```python
from build123d import *

# Parameters (mm, degrees)
BOSS_EXTRUDE1_DEPTH  = 6.604
MOVE_FACE1_DEPTH     = 6.604
MOVE_FACE1_2_DEPTH   = 6.604
BOSS_EXTRUDE2_DEPTH  = 21.59
BOSS_EXTRUDE3_REACH  = 135.651
FILLET1_R            = 12.7
BOSS_EXTRUDE4_DEPTH  = 4.0259
MIRROR3_COPY_1_DEPTH = 4.0259
SKETCH13_R           = 6.35
CUT_EXTRUDE1_DEPTH   = 110.931012164
SKETCH9_R            = 47.625
SKETCH9_R_2          = 43.434
BOSS_EXTRUDE7_DEPTH  = 1.27
CUT_EXTRUDE2_START   = -5.08
SKETCH15_R           = 43.434
CUT_EXTRUDE2_DEPTH   = 5.08
SKETCH16_R           = 15.24
CUT_EXTRUDE3_DEPTH   = 2.54
SKETCH17_R           = 15.24
BOSS_EXTRUDE8_DEPTH  = 11.2395
SKETCH18_R           = 12.7
CUT_EXTRUDE4_DEPTH   = 6.35


# Read off the part's stored shape, not the designer's step: Move Face1
with BuildPart() as part:
    # Sketch1 → Boss-Extrude1 (new body)
    with BuildSketch(Plane(origin=(0, 0, 0), x_dir=(1, 0, 0), z_dir=(0, 1, 0))):
        with BuildLine():
            Line((0, 27.051), (0, -27.051))
            Line((0, -27.051), (5.969168013, -48.482817353))
            ThreePointArc((5.969168013, -48.482817353), (14.05820124, -57.663213719), (26.276846155, -57.017572631))
            Line((26.276846155, -57.017572631), (47.13309789, -51.810845761))
            ThreePointArc((47.13309789, -51.810845761), (58.8645, -50.8), (70.59590211, -51.810845761))
            Line((70.59590211, -51.810845761), (91.452153845, -57.017572631))
            ThreePointArc((91.452153845, -57.017572631), (103.67079876, -57.663213719), (111.759831987, -48.482817353))
            Line((111.759831987, -48.482817353), (117.729, -27.051))
            Line((117.729, -27.051), (117.729, 27.051))
            Line((117.729, 27.051), (111.759831987, 48.482817353))
            ThreePointArc((111.759831987, 48.482817353), (103.67079876, 57.663213719), (91.452153845, 57.017572631))
            Line((91.452153845, 57.017572631), (70.59590211, 51.810845761))
            ThreePointArc((70.59590211, 51.810845761), (58.8645, 50.8), (47.13309789, 51.810845761))
            Line((47.13309789, 51.810845761), (26.276846155, 57.017572631))
            ThreePointArc((26.276846155, 57.017572631), (14.05820124, 57.663213719), (5.969168013, 48.482817353))
            Line((5.969168013, 48.482817353), (0, 27.051))
        make_face()
    extrude(amount=BOSS_EXTRUDE1_DEPTH)

    # Move Face1 outline → Move Face1 (cut)
    with BuildSketch(Plane(origin=(0, 0, 0), x_dir=(1, 0, 0), z_dir=(0, 1, 0))):
        with BuildLine():
            ThreePointArc((11.73140211, -51.810845761), (9.381670874, -51.444731901), (7.020658859, -51.160305269))
            ThreePointArc((7.020658859, -51.160305269), (15.412744455, -58.152404227), (26.276846155, -57.017572631))
            Line((26.276846155, -57.017572631), (29.43225, -56.229831564))
            Line((29.43225, -56.229831564), (11.73140211, -51.810845761))
        make_face()
        with BuildLine():
            ThreePointArc((26.276846155, 57.017572631), (15.412744455, 58.152404227), (7.020658859, 51.160305269))
            ThreePointArc((7.020658859, 51.160305269), (9.381670874, 51.444731901), (11.73140211, 51.810845761))
            Line((11.73140211, 51.810845761), (29.43225, 56.229831564))
            Line((29.43225, 56.229831564), (26.276846155, 57.017572631))
        make_face()
        with BuildLine():
            ThreePointArc((52.895331987, -48.482817353), (52.438308346, -49.848549416), (51.843841141, -51.160305269))
            ThreePointArc((51.843841141, -51.160305269), (61.242225011, -50.841231235), (70.59590211, -51.810845761))
            Line((70.59590211, -51.810845761), (91.452153845, -57.017572631))
            ThreePointArc((91.452153845, -57.017572631), (103.67079876, -57.663213719), (111.759831987, -48.482817353))
            Line((111.759831987, -48.482817353), (117.729, -27.051))
            Line((117.729, -27.051), (117.729, 27.051))
            Line((117.729, 27.051), (111.759831987, 48.482817353))
            ThreePointArc((111.759831987, 48.482817353), (103.67079876, 57.663213719), (91.452153845, 57.017572631))
            Line((91.452153845, 57.017572631), (70.59590211, 51.810845761))
            ThreePointArc((70.59590211, 51.810845761), (61.242225011, 50.841231235), (51.843841141, 51.160305269))
            ThreePointArc((51.843841141, 51.160305269), (52.438308346, 49.848549416), (52.895331987, 48.482817353))
            Line((52.895331987, 48.482817353), (58.8645, 27.051))
            Line((58.8645, 27.051), (58.8645, -27.051))
            Line((58.8645, -27.051), (52.895331987, -48.482817353))
        make_face()
    extrude(amount=MOVE_FACE1_DEPTH, mode=Mode.SUBTRACT)

    # Move Face1 2 outline → Move Face1 2 (add)
    with BuildSketch(Plane(origin=(0, 0, 0), x_dir=(1, 0, 0), z_dir=(0, 1, 0))):
        with BuildLine():
            Line((-58.8645, -27.051), (-52.895331987, -48.482817353))
            ThreePointArc((-52.895331987, -48.482817353), (-44.80629876, -57.663213719), (-32.587653845, -57.017572631))
            Line((-32.587653845, -57.017572631), (-11.73140211, -51.810845761))
            ThreePointArc((-11.73140211, -51.810845761), (-2.377725011, -50.841231235), (7.020658859, -51.160305269))
            ThreePointArc((7.020658859, -51.160305269), (6.426191654, -49.848549416), (5.969168013, -48.482817353))
            Line((5.969168013, -48.482817353), (0, -27.051))
            Line((0, -27.051), (0, 27.051))
            Line((0, 27.051), (5.969168013, 48.482817353))
            ThreePointArc((5.969168013, 48.482817353), (6.426191654, 49.848549416), (7.020658859, 51.160305269))
            ThreePointArc((7.020658859, 51.160305269), (-2.377725011, 50.841231235), (-11.73140211, 51.810845761))
            Line((-11.73140211, 51.810845761), (-32.587653845, 57.017572631))
            ThreePointArc((-32.587653845, 57.017572631), (-44.80629876, 57.663213719), (-52.895331987, 48.482817353))
            Line((-52.895331987, 48.482817353), (-58.8645, 27.051))
            Line((-58.8645, 27.051), (-58.8645, -27.051))
        make_face()
        with BuildLine():
            Line((47.13309789, -51.810845761), (29.43225, -56.229831564))
            Line((29.43225, -56.229831564), (32.587653845, -57.017572631))
            ThreePointArc((32.587653845, -57.017572631), (43.451755545, -58.152404227), (51.843841141, -51.160305269))
            ThreePointArc((51.843841141, -51.160305269), (49.482829126, -51.444731901), (47.13309789, -51.810845761))
        make_face()
        with BuildLine():
            Line((32.587653845, 57.017572631), (29.43225, 56.229831564))
            Line((29.43225, 56.229831564), (47.13309789, 51.810845761))
            ThreePointArc((47.13309789, 51.810845761), (49.482829126, 51.444731901), (51.843841141, 51.160305269))
            ThreePointArc((51.843841141, 51.160305269), (43.451755545, 58.152404227), (32.587653845, 57.017572631))
        make_face()
    extrude(amount=MOVE_FACE1_2_DEPTH)

    # Sketch5 → Boss-Extrude2 (add)
    with BuildSketch(Plane(origin=(58.8645, 0, 0), x_dir=(0, 0, -1), z_dir=(1, 0, 0))):
        with BuildLine():
            Line((-23.199811166, 50.623289797), (-27.051, 6.604))
            Line((-27.051, 6.604), (27.051, 6.604))
            Line((27.051, 6.604), (23.199811166, 50.623289797))
            ThreePointArc((23.199811166, 50.623289797), (0, 71.882), (-23.199811166, 50.623289797))
        make_face()
    boss_extrude2 = extrude(amount=-BOSS_EXTRUDE2_DEPTH)

    # Mirror1: Boss-Extrude2 across plane
    add(boss_extrude2.mirror(Plane(origin=(0, 0, 0), x_dir=(0, 0, 1), z_dir=(1, 0, 0))))

    # Sketch7 → Boss-Extrude3 (add, up to next)
    with BuildSketch(Plane.ZY.offset(-37.2745), mode=Mode.PRIVATE) as boss_extrude3_sk1:
        Polygon((-27.051, 6.604), (27.051, 6.604), (0, 25.654), align=None)
    boss_extrude3_tool1 = extrude(boss_extrude3_sk1.sketch, amount=BOSS_EXTRUDE3_REACH, mode=Mode.PRIVATE) - part.part
    add(boss_extrude3_tool1.solids().sort_by_distance((37.2745, 12.954, 0))[0])

    # Fillet1
    fillet1_edges = [part.edges().sort_by_distance(p)[0] for p in [
        (0, 25.654, 0),
    ]]
    fillet(fillet1_edges, radius=FILLET1_R)

    # Sketch8 → Boss-Extrude4 (add)
    with BuildSketch(Plane(origin=(0, 6.604, 0), x_dir=(1, 0, 0), z_dir=(0, 1, 0))):
        with BuildLine():
            Line((-57.546161193, -27.051), (-51.671898381, -48.142067867))
            ThreePointArc((-51.671898381, -48.142067867), (-44.239742404, -56.523444134), (-33.059468887, -55.82638267))
            ThreePointArc((-33.059468887, -55.82638267), (-30.556113123, -54.093687416), (-28.541750469, -51.810845761))
            ThreePointArc((-28.541750469, -51.810845761), (-27.780193276, -37.622311234), (-37.2745, -27.051))
            Line((-37.2745, -27.051), (-57.546161193, -27.051))
        make_face()
    boss_extrude4 = extrude(amount=BOSS_EXTRUDE4_DEPTH)

    # Mirror2: Boss-Extrude4 across plane
    add(boss_extrude4.mirror(Plane(origin=(0, 0, 0), x_dir=(0, 0, 1), z_dir=(1, 0, 0))))

    # Mirror3: Boss-Extrude4 across plane
    add(boss_extrude4.mirror(Plane.XY))

    # Mirror3 copy 1 sketch → Mirror3 copy 1 (add)
    with BuildSketch(Plane(origin=(0, 6.604, 0), x_dir=(-1, 0, 0), z_dir=(0, 1, 0))):
        with BuildLine():
            Line((-57.546161193, -27.051), (-51.671898381, -48.142067867))
            ThreePointArc((-51.671898381, -48.142067867), (-44.239742404, -56.523444134), (-33.059468887, -55.82638267))
            ThreePointArc((-33.059468887, -55.82638267), (-30.556113123, -54.093687416), (-28.541750469, -51.810845761))
            ThreePointArc((-28.541750469, -51.810845761), (-27.780193276, -37.622311234), (-37.2745, -27.051))
            Line((-37.2745, -27.051), (-57.546161193, -27.051))
        make_face()
    extrude(amount=MIRROR3_COPY_1_DEPTH)

    # Sketch13 → Cut-Extrude1 (cut, through all)
    with BuildSketch(Plane(origin=(0, 0, 0), x_dir=(-1, 0, 0), z_dir=(0, -1, 0))):
        with Locations(Location((39.240708081, -45.97811401, 0), (0, 0, 90))):
            Circle(SKETCH13_R)
        with Locations(Location((-38.229291919, -45.81936236, 0), (0, 0, 90))):
            Circle(SKETCH13_R)
        with Locations(Location((-37.975496477, 46.39533764, 0), (0, 0, 90))):
            Circle(SKETCH13_R)
        with Locations(Location((39.494503523, 46.12740723, 0), (0, 0, 90))):
            Circle(SKETCH13_R)
    extrude(amount=-CUT_EXTRUDE1_DEPTH, mode=Mode.SUBTRACT)

    # Sketch9 → Boss-Extrude7 (add)
    with BuildSketch(Plane.XZ):
        with Locations(Location((0, 0, 0), (0, 0, 90))):
            Circle(SKETCH9_R)
        with Locations(Location((0, 0, 0), (0, 0, 270))):
            Circle(SKETCH9_R_2, mode=Mode.SUBTRACT)
    extrude(amount=BOSS_EXTRUDE7_DEPTH)

    # Sketch15 → Cut-Extrude2 (cut)
    with BuildSketch(Plane.XZ.offset(CUT_EXTRUDE2_START)):
        with Locations(Location((0, 0, 0), (0, 0, 270))):
            Circle(SKETCH15_R)
    extrude(amount=CUT_EXTRUDE2_DEPTH, mode=Mode.SUBTRACT)

    # Sketch16 → Cut-Extrude3 (cut)
    with BuildSketch(Plane(origin=(58.8645, 0, 0), x_dir=(0, 0, -1), z_dir=(1, 0, 0))):
        with Locations((0, 48.593569324)):
            Circle(SKETCH16_R)
    cut_extrude3 = extrude(amount=-CUT_EXTRUDE3_DEPTH, mode=Mode.SUBTRACT)

    # Sketch17 → Boss-Extrude8 (add)
    with BuildSketch(Plane.ZY.offset(-37.2745)):
        with Locations(Location((0, 48.593569324, 0), (0, 0, 180))):
            Circle(SKETCH17_R)
    boss_extrude8 = extrude(amount=BOSS_EXTRUDE8_DEPTH)

    # Sketch18 → Cut-Extrude4 (cut)
    with BuildSketch(Plane.ZY.offset(-26.035)):
        with Locations((0, 48.593569324)):
            Circle(SKETCH18_R)
    cut_extrude4 = extrude(amount=-CUT_EXTRUDE4_DEPTH, mode=Mode.SUBTRACT)

    # Mirror4: Cut-Extrude3, Boss-Extrude8, Cut-Extrude4 across plane
    add(cut_extrude3.mirror(Plane(origin=(0, 0, 0), x_dir=(0, 0, 1), z_dir=(1, 0, 0))), mode=Mode.SUBTRACT)
    add(boss_extrude8.mirror(Plane(origin=(0, 0, 0), x_dir=(0, 0, 1), z_dir=(1, 0, 0))))
    add(cut_extrude4.mirror(Plane(origin=(0, 0, 0), x_dir=(0, 0, 1), z_dir=(1, 0, 0))), mode=Mode.SUBTRACT)


solid = part.part
```
Geometry check sheet. Reference: the model listing, model coordinates, mm. A direction names the side the tool comes from. Give positions to 0.01 mm unless a question says otherwise; leave off trailing zeros. Order: outer loops, then holes, each group sorted by start corner. A loop starts at its lowest first (then second) coordinate and runs counter-clockwise, first axis right, second up. Notation, with made-up numbers: (59.25, 65) -> (113.25, 65) arc R19 cw to (113.25, 79) -> close; hole circle Ø2 at (69, -0.5). An arc over 180 degrees is marked (long way). Write each question's results on one line, items separated by ' | '. Start each with the question number.
(1) Sectioned sample at C-C (z = 31). Enter the section's corners in (x, y), plus the area to 3 significant figures.
(2) Access from +Z, -Z, +X, -X, +Y, -Y to the whole of each face (thin tool, end or side, straight path). Record for faces 1 (the face through (-22.31, 3.26, 54.45)), 2 (the face through (42, 10.63, 39)), 3 (the face through (-30.588, 8.589, 54.122)), 4 (the face through (-31.733, 33.483, 1.984)), 5 (the face through (56.324, 49, 0)).
(3) Gauge pin test, flat ends, axial feed: P1, Ø1.5, axis at x = 22, z = 26, coming from the -Y side; P2, Ø24.5, axis at y = 48.59, z = 0, coming from the -X side; P3, Ø8, axis at x = 8.5, y = 6.5, coming from the -Z side; P4, Ø7.5, axis at x = 38.23, z = 45.82, coming from the -Y side. Record the tip position at first contact, or that the pin passes through.
(4) Mould release check, pull along Y, two halves, no side actions. Record for faces 6 (the face through (37.274, 32, 0)), 7 (the face through (-5, 0, -48)), 8 (the face through (-1, 6.604, 39)), 9 (the face through (-44.39, 8.59, 56.46)): pulls with the +Y half, pulls with the -Y half, needs draft (parallel to the pull), parting line crosses it, or undercut.
(5) Sectioned sample at A-A (x = 0). Enter the section's corners in (y, z) (3 decimals).
(6) Scan lines: line 1 (X direction, y = 9, z = -25.5); line 2 (X direction, y = 57, z = 0.5) (1 decimal); line 3 (Y direction, x = 57.8, z = 0). Record each from-to range of solid material in increasing order.
(7) Sectioned sample at D-D (x = -17). Enter the section's corners in (y, z).
Answer below:
1) outline: (-57.76, 0) -> (-36.15, 0) -> (-36.15, -1.27) -> (-30.42, -1.27) -> (-30.42, 5.08) -> (30.42, 5.08) -> (30.42, -1.27) -> (36.15, -1.27) -> (36.15, 0) -> (57.76, 0) -> (57.76, 6.6) -> (56.45, 6.6) -> (56.45, 10.63) -> (31.84, 10.63) -> (31.84, 6.6) -> (-31.84, 6.6) -> (-31.84, 10.63) -> (-56.45, 10.63) -> (-56.45, 6.6) -> (-57.76, 6.6) -> close | area: 667 mm2
2) face 1: +Z, +Y, -Y | face 2: +Z, +X, -X, +Y | face 3: +Z, +Y | face 4: none | face 5: +X
3) P1: y = 5.08 | P2: x = -56.32 | P3: z = -52 | P4: through
4) face 6: undercut | face 7: pulls with the -Y half | face 8: pulls with the +Y half | face 9: needs draft
5) outline: (-1.27, -47.625) -> (0, -47.625) -> (0, -50.8) -> (6.604, -50.8) -> (6.604, -27.051) -> (20.504, -7.312) arc R12.7 ccw to (20.504, 7.312) -> (6.604, 27.051) -> (6.604, 50.8) -> (0, 50.8) -> (0, 47.625) -> (-1.27, 47.625) -> (-1.27, 43.434) -> (5.08, 43.434) -> (5.08, -43.434) -> (-1.27, -43.434) -> close
6) line 1: -58.86 to -37.27, 37.27 to 58.86 | line 2: -56.3 to -32.4, 32.4 to 56.3 | line 3: 0 to 33.35, 63.83 to 71.88
7) outline: (-1.27, -44.49) -> (0, -44.49) -> (0, -53.13) -> (6.6, -53.13) -> (6.6, -27.05) -> (20.5, -7.31) arc R12.7 ccw to (20.5, 7.31) -> (6.6, 27.05) -> (6.6, 53.13) -> (0, 53.13) -> (0, 44.49) -> (-1.27, 44.49) -> (-1.27, 39.97) -> (5.08, 39.97) -> (5.08, -39.97) -> (-1.27, -39.97) -> close
